Autodesk Inventor part; units mm, degrees
ref_plane "YZ Plane" through (0, 0, 0) normal (1, 0, 0) x (0, 1, 0)
ref_plane "XZ Plane" through (0, 0, 0) normal (0, 1, 0) x (-1, 0, 0)
ref_plane "XY Plane" through (0, 0, 0) normal (0, 0, 1) x (1, 0, 0)
sketch "Sketch1" plane through (0, 0, 0) normal (0, 1, 0) x (-1, 0, 0)
  circle A0 centre (0, 0) radius 21.25
  circle A1 centre (0, 0) radius 18.25
  point P0 (0, 18.25)
  point P1 (15.676, 9.3448)
  dimension "d0" = 42.5
  dimension "d3" = 3
  dimension "d4" = 59.2
extrude "Extrusion1" add sketch "Sketch1" along normal blind 2 contours A0 | A1
hole "Hole1" at (0, 0, 18.25) at (-15.676, 0, 9.3448) direction (0, 1, 0) diameter 3 depth 8 tip angle 118
hole "Hole2" at (0, 0, 0) direction (0, 1, 0) diameter 5 depth 8 tip angle 118
properties part number "RotatoryDisk"
For this review, take the finished solid that the model builds, in its own axes (mm). Give positions to 0.01 mm unless a question says otherwise; leave off trailing zeros. Order: outer loops, then holes, each group sorted by start corner. A loop starts at its lowest first (then second) coordinate and runs counter-clockwise, first axis right, second up.
1) Insertion check: pin 1 (1 mm diameter, centred on x = 12, y = 1.5, fed in from +Z); pin 2 (1 mm diameter, centred on x = 11, y = 1.5, fed in from -Z). Each pin has a flat end and moves straight along its axis. Give the tip position at first contact, or say it passes through.
2) Take a section at D-D (z = 18.25). Give the boundary of the cut face in (x, y), then the cut area to 3 significant figures.
3) Wall thickness on line 1 (Z direction, x = 0, y = 0.55); line 2 (Z direction, x = 0.5, y = 1.35); line 3 (X direction, y = 1.8, z = 10): over which ranges is each line inside the solid? List them lowest first.
4) Take a section at A-A (x = 0). Give the boundary of the cut face in (y, z), then the cut area to 3 significant figures.
5) Take a section at C-C (y = 0.75). Give the boundary of the cut face in (x, z), then the cut area to 3 significant figures.
6) Take a section at B-B (z = 0). Give the boundary of the cut face in (x, y).
7) The part is to be moulded in two halves that separate along Z. For faces 1 (the face through (-15.1, 1.01, 7.96)), 2 (the face through (0, 2, -4)), 3 (the face through (16.863, 0.986, 12.93)), say which applies: released by +Z, released by -Z, zero draft, split by the parting line, or undercut.
Derived:
1. pin 1: stops at z = 17.87
1. pin 2: stops at z = -18.47
2. outline: (-10.89, 0) - (-1.5, 0) - (-1.5, 2) - (-10.89, 2) - close; (1.5, 0) - (10.89, 0) - (10.89, 2) - (1.5, 2) - close
2. area: 37.5 mm2
3. line 1: z = -21.25 to -2.5, 2.5 to 16.75, 19.75 to 21.25
3. line 2: z = -21.24 to -2.45, 2.45 to 16.84, 19.66 to 21.24
3. line 3: x = -18.75 to -17.03, -14.33 to 18.75
4. outline: (0, -21.25) - (2, -21.25) - (2, -2.5) - (0, -2.5) - close; (0, 2.5) - (2, 2.5) - (2, 16.75) - (0, 16.75) - close; (0, 19.75) - (2, 19.75) - (2, 21.25) - (0, 21.25) - close
4. area: 69.0 mm2
5. outline: circle Ø42.5 at (0, 0); hole circle Ø3 at (-15.68, 9.34); hole circle Ø5 at (0, 0); hole circle Ø3 at (0, 18.25)
5. area: 1,380 mm2
6. outline: (-21.25, 0) - (-2.5, 0) - (-2.5, 2) - (-21.25, 2) - close; (2.5, 0) - (21.25, 0) - (21.25, 2) - (2.5, 2) - close
7. face 1: undercut
7. face 2: zero draft
7. face 3: split by the parting line
